Verification items for the finished model (mm, model axes). A direction names the side the tool comes from. Give positions to 0.01 mm unless a question says otherwise; leave off trailing zeros. Use one line per item in the form item = value. Start each with the question number.
(1) Scan lines: L1, parallel to Z at x = 0, y = 0.1 (3 decimals); L2, parallel to Z at x = 0, y = -1 (1 decimal); L3, parallel to X at y = -1.3, z = -1.75. Record each from-to range of solid material in increasing order.
(2) Set-up check for faces 1 (the face through (-0.461, -3.375, 3.513)), 2 (the face through (-3.78, -1.57, -2.9)), 3 (the face through (0.461, 0.2, 3.513)): record each of +Z, -Z, +X, -X, +Y, -Y from which the full face is reachable in a straight line by a thin tool's end or side.
(3) Depth check by flat-ended pin: pin 1 Ø2 at (x, y) = (3.5, -1.5) entering from -Z; pin 2 Ø4 at (x, z) = (0, 0) entering from -Y. Enter the tip coordinate at first touch or a pass-through.
from build123d import *

# Parameters (mm, degrees)
F0_R     = 4.7625
F0_R_2   = 3.175
F1_DEPTH = 3.175
F2_R     = 3.5433
F2_R_2   = 3.175
F3_DEPTH = 0.4064
F4_R     = 3.5433
F4_R_2   = 3.175
F5_DEPTH = 0.4064
F6_SIZE  = 0.254


with BuildPart() as f1:
    # F0 (on Front) → F1 (new body)
    with BuildSketch(Plane.XZ):
        Circle(F0_R)
        Circle(F0_R_2, mode=Mode.SUBTRACT)
    extrude(amount=F1_DEPTH)

    # F2 (on face) → F3 (join)
    with BuildSketch(Plane.XZ.offset(3.175)):
        Circle(F2_R)
        Circle(F2_R_2, mode=Mode.SUBTRACT)
    extrude(amount=F3_DEPTH)

    # F4 (on face) → F5 (join)
    with BuildSketch(Plane(origin=(0, 0, 0), x_dir=(-1, 0, 0), z_dir=(0, 1, 0))):
        Circle(F4_R)
        Circle(F4_R_2, mode=Mode.SUBTRACT)
    extrude(amount=F5_DEPTH)

    # F6
    f6_edges = [f1.edges().sort_by_distance(p)[0] for p in [
        (-4.7625, -3.175, 0),
        (-4.7625, 0, 0),
    ]]
    chamfer(f6_edges, length=F6_SIZE)


solid = f1.part
Completed:
q1.L1 = -3.543 to -3.175, 3.175 to 3.543
q1.L2 = -4.8 to -3.2, 3.2 to 4.8
q1.L3 = -4.43 to -2.65, 2.65 to 4.43
q2.face_1 = -Y
q2.face_2 = +Y, -Y
q2.face_3 = +Y
q3.pin_1 = -4.05
q3.pin_2 = through
